from build123d import *

# Parameters (mm, degrees)
F0_W     = 31
F0_H     = 740
F0_W_2   = 9
F0_W_3   = 71
F0_W_4   = 35.5
F1_DEPTH = 15
F2_DEPTH = 10


with BuildPart() as f1:
    # F0 (on Top) → F1 (new body)
    with BuildSketch(Plane.XY):
        with Locations((180, 0)):
            Rectangle(F0_W, F0_H)
        with Locations((160, 0)):
            Rectangle(F0_W_2, F0_H)
        with Locations((200, 0)):
            Rectangle(F0_W_2, F0_H)
        with Locations((120, 0)):
            Rectangle(F0_W_3, F0_H)
        with Locations((80, 0)):
            Rectangle(F0_W_2, F0_H)
        with Locations((60, 0)):
            Rectangle(F0_W, F0_H)
        with Locations((40, 0)):
            Rectangle(F0_W_2, F0_H)
        with Locations((222.25, 0)):
            Rectangle(F0_W_4, F0_H)
        with Locations((17.75, 0)):
            Rectangle(F0_W_4, F0_H)
    extrude(amount=-F1_DEPTH)

    # F0 (on Top) → F2 (cut)
    with BuildSketch(Plane.XY):
        with Locations((40, 0)):
            Rectangle(F0_W_2, F0_H)
        with Locations((80, 0)):
            Rectangle(F0_W_2, F0_H)
        with Locations((160, 0)):
            Rectangle(F0_W_2, F0_H)
        with Locations((200, 0)):
            Rectangle(F0_W_2, F0_H)
    extrude(amount=-F2_DEPTH, mode=Mode.SUBTRACT)

    # F3: F1 across face


with BuildPart() as f1_1:
    add(f1.part)
    add(f1.part.mirror(Plane(origin=(0, 0, -7.5), x_dir=(0, -1, 0), z_dir=(-1, 0, 0))))


solid = f1_1.part
For this review, take the finished solid that the model builds, in its own axes (mm). Round coordinates to 2 decimals unless told otherwise and drop trailing zeros. Put each result on its own line as item: value. Start each with the question number.
1. Consider section A-A on z = -6.25. State how many separate pieces and enclosed holes the cut face has, plus the area to 3 significant figures.
2. For probe 1 along Z at (x, y) = (-38, 283), list the stretches that pass through material, from the lowest coordinate up. Write a range as [from, to].
3. Insertion check: P1, Ø4.5, axis at x = -80.5, y = 46.5, coming from the +Z side; P2, Ø10, axis at x = 82, y = 148, coming from the +Z side. Each pin has a flat end and moves straight along its axis. Give the tip position at first contact, or say it passes through.
Result sheet:
1. separate pieces: 9
1. enclosed holes: 0
1. area: 302,000 mm^2
2. probe 1: [-15, -10]
3. P1: z = -10
3. P2: z = 0
